Read the model definition and answer for the solid it produces. Units are mm, in the model's axes. A direction names the side the tool comes from. Round coordinates to 2 decimals unless told otherwise and drop trailing zeros. Write each loop counter-clockwise with the first axis right and the second up, starting at its lowest first coordinate (ties: lowest second). Pieces come first, ordered by that corner, then holes. Notation, with made-up numbers: (75.5, 18) - (80.5, 18) arc R30 ccw to (80.5, 55) - close; hole circle Ø10 at (81, -22). An arc over 180 degrees is marked (long way). Use one line per item in the form item = value. Start each with the question number.
1) The part is cut by section D-D, the plane x = -14. Give the vertices of the cut face in (y, z) (3 decimals).
2) Consider line 1 along Z through (x, y) = (6, 44) (3 decimals); line 2 along X through (y, z) = (28, 2.5). Determine where each line is inside the solid, lowest interval first. Write a range as from..to.
3) The part is cut by section C-C, the plane z = 11.5. Give the vertices of the cut face in (x, y), plus the area to 3 significant figures.
4) For a pull along Y with two mould halves and no side action, classify faces 1 (the face through (-19.05, 13, -5)), 2 (the face through (-1.356, 21.19, 6.53)), 3 (the face through (13, 57.15, -5)) as released by +Y, released by -Y, zero draft, split by the parting line, or undercut.
5) The part is cut by section A-A, the plane x = 10. Give the vertices of the cut face in (y, z) (3 decimals), plus the area to 3 significant figures.
6) Each of these flat-tipped pins is pushed along its axis until it touches: pin 1 (2.5 mm diameter, centred on y = 46.5, z = -4, fed in from -X); pin 2 (5 mm diameter, centred on x = -1.5, y = 46, fed in from -Z); pin 3 (8 mm diameter, centred on x = -3.5, y = 17, fed in from +Z) (3 decimals); pin 4 (2.5 mm diameter, centred on x = -14, z = -4.5, fed in from +Y). Where does it stop, or does it pass through?
7) For faces 4 (the face through (-14, 25.4, -5)), 5 (the face through (3, 29, -6.35)), determine the directions among +Z, -Z, +X, -X, +Y, -Y from which every point of the face is accessible in a straight line to the end or side of a thin tool.
8) The part is cut by section B-B, the plane y = 18. Give the vertices of the cut face in (x, z) (3 decimals), plus the area to 3 significant figures.
from build123d import *

# Parameters (mm, degrees)
F0_R     = 6.35
F1_DEPTH = 22.86
F2_DEPTH = 3.175
F3_ANGLE = 180


with BuildPart() as f1:
    # F0 (on Top) → F1 (new body)
    with BuildSketch(Plane.XY):
        with Locations((-4.509694, 23.622)):
            Circle(F0_R)
    extrude(amount=-F1_DEPTH)

    # F0 (on Top) → F2 (join)
    with BuildSketch(Plane.XY):
        with BuildLine():
            Line((0, 57.15), (-25.4, 57.15))
            Line((-25.4, 57.15), (-25.4, 34.925))
            ThreePointArc((-25.4, 34.925), (-15.170704, 10.229296), (9.525, 0))
            Line((9.525, 0), (19.05, 0))
            Line((19.05, 0), (19.05, 25.4))
            Line((19.05, 25.4), (9.525, 25.4))
            ThreePointArc((9.525, 25.4), (2.789808, 28.189808), (0, 34.925))
            Line((0, 34.925), (0, 57.15))
        make_face()
        with Locations((-4.509694, 23.622)):
            Circle(F0_R, mode=Mode.SUBTRACT)
    extrude(amount=-F2_DEPTH)


with BuildPart() as f1_1:
    # F3: moved
    add(f1.part.rotate(Axis((0, 46.0375, -3.175), (0, 1, 0)), F3_ANGLE))


solid = f1_1.part
Geometry results:
q1.outline = (0, -6.35) - (25.4, -6.35) - (25.4, -3.175) - (0, -3.175) - close
q2.line_1 = -6.35..-3.175
q2.line_2 = -0.09..9.11
q3.outline = circle Ø12.7 at (4.51, 23.62)
q3.area = 127 mm2
q4.face_1 = zero draft
q4.face_2 = split by the parting line
q4.face_3 = released by +Y
q5.outline = (5.968, -6.35) - (57.15, -6.35) - (57.15, -3.175) - (26.812, -3.175) - (26.812, 16.51) - (20.432, 16.51) - (20.432, -3.175) - (5.968, -3.175) - close
q5.area = 288 mm2
q6.pin_1 = 0
q6.pin_2 = -6.35
q6.pin_3 = -3.175
q6.pin_4 = 25.4
q7.face_4 = +Z, -Z, -X, +Y
q7.face_5 = -Z, +X, -X, +Y, -Y
q8.outline = (-19.05, -6.35) - (21.025, -6.35) - (21.025, -3.175) - (7.462, -3.175) - (7.462, 16.51) - (1.557, 16.51) - (1.557, -3.175) - (-19.05, -3.175) - close
q8.area = 243 mm2
